Geometry check sheet. Reference: drawing and pictorial views, mm from the part's lowest x, y, z. A direction names the side the tool comes from. Round coordinates to 2 decimals unless told otherwise and drop trailing zeros. Order: outer loops, then holes, each group sorted by start corner. A loop starts at its lowest first (then second) coordinate and runs counter-clockwise, first axis right, second up.
(1) Sectioned sample at A-A, the plane y = 15.24. Enter the section's corners in (x, z) (3 decimals), and give its area (3 significant figures).
(2) Sectioned sample at D-D, the plane y = 5. Enter the section's corners in (x, z), and give its area (3 significant figures).
(3) Sectioned sample at B-B, the plane z = 40.5. Enter the section's corners in (x, y), and give its area (3 significant figures).
(4) Sectioned sample at C-C, the plane x = 3. Enter the section's corners in (y, z) (3 decimals), and give its area (3 significant figures).
(5) Thickness scan on probe 1 along Y at (x, z) = (7.5, 53.34) (3 decimals); probe 2 along Z at (x, y) = (2.25, 14.5) (1 decimal); probe 3 along Y at (x, z) = (3, 15.24). Record the ranges inside material, lowest first.
(6) Tool access check on the marked faces 4 and 5. Record the directions out of +Z, -Z, +X, -X, +Y, -Y that give a thin tool (end or side, any length) a straight path to the whole face; none if there is none.
(7) Depth check by flat-ended pin: pin 1 (3 mm diameter, centred on x = 2.5, y = 13, fed in from -Z); pin 2 (3 mm diameter, centred on x = 5.5, y = 5.5, fed in from +Z); pin 3 (5 mm diameter, centred on x = 4, y = 25, fed in from +Z). Enter the tip coordinate at first touch or a pass-through.
(8) Mould release check, pull along Y, two halves, no side actions. Record for the marked faces 1, 2 and 3: released by +Y, released by -Y, zero draft, split by the parting line, or undercut.
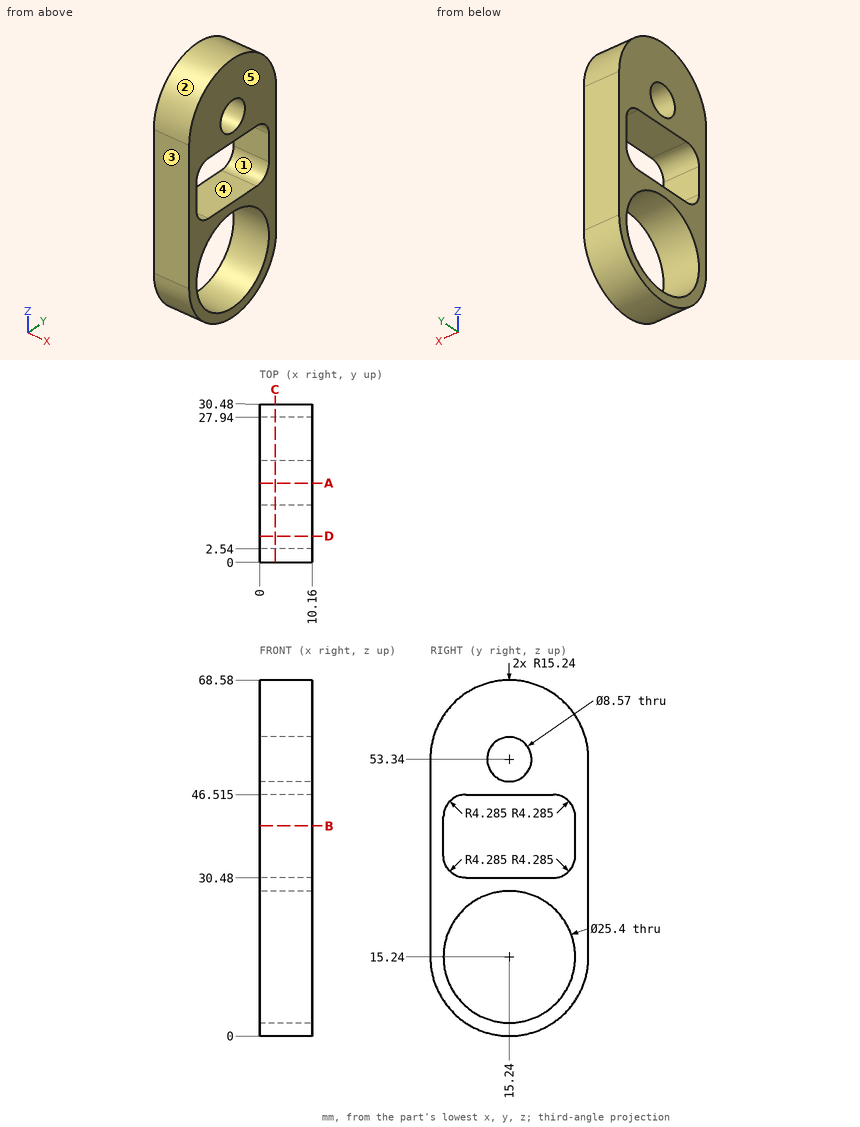
Derived:
1. outline: (0, 0) - (10.16, 0) - (10.16, 2.54) - (0, 2.54) - close; (0, 27.94) - (10.16, 27.94) - (10.16, 30.48) - (0, 30.48) - close; (0, 46.515) - (10.16, 46.515) - (10.16, 49.055) - (0, 49.055) - close; (0, 57.625) - (10.16, 57.625) - (10.16, 68.58) - (0, 68.58) - close
1. area: 189 mm2
2. outline: (0, 3.95) - (10.16, 3.95) - (10.16, 7.73) - (0, 7.73) - close; (0, 22.75) - (10.16, 22.75) - (10.16, 30.89) - (0, 30.89) - close; (0, 46.11) - (10.16, 46.11) - (10.16, 64.63) - (0, 64.63) - close
2. area: 309 mm2
3. outline: (0, 0) - (10.16, 0) - (10.16, 2.54) - (0, 2.54) - close; (0, 27.94) - (10.16, 27.94) - (10.16, 30.48) - (0, 30.48) - close
3. area: 51.6 mm2
4. outline: (0, 15.24) arc R15.24 ccw to (30.48, 15.24) - (30.48, 53.34) arc R15.24 ccw to (0, 53.34) - close; hole circle Ø25.4 at (15.24, 15.24); hole (2.54, 34.765) arc R4.285 ccw to (6.825, 30.48) - (23.655, 30.48) arc R4.285 ccw to (27.94, 34.765) - (27.94, 42.23) arc R4.285 ccw to (23.655, 46.515) - (6.825, 46.515) arc R4.285 ccw to (2.54, 42.23) - close; hole circle Ø8.57 at (15.24, 53.34)
4. area: 935 mm2
5. probe 1: y = 0 to 10.955, 19.525 to 30.48
5. probe 2: z = 0 to 2.6, 27.9 to 30.5, 46.5 to 49.1, 57.6 to 68.6
5. probe 3: y = 0 to 2.54, 27.94 to 30.48
6. face 4: +X, -X
6. face 5: +Z, -Z, +X, +Y, -Y
7. pin 1: stops at z = 0.02
7. pin 2: stops at z = 66.16
7. pin 3: stops at z = 66.74
8. face 1: undercut
8. face 2: split by the parting line
8. face 3: released by -Y
